from build123d import *

# Parameters (mm, degrees)
F0_W     = 75
F0_H     = 100
F0_R     = 4
F1_DEPTH = 2
F2_R     = 1.584077
F2_R_2   = 1.709737
F2_R_3   = 1.732285
F2_R_4   = 1.739733
F2_R_5   = 1.525849
F2_R_6   = 1.456457
F2_R_7   = 1.732284
F2_R_8   = 1.660922
F2_R_9   = 1.609722
F2_R_10  = 1.290227
F2_R_11  = 1.875683
F2_R_12  = 1.517347
F2_R_13  = 1.874836
F2_R_14  = 1.624248
F2_R_15  = 1.319184
F2_R_16  = 1.584076
F2_R_17  = 1.326308
F2_R_18  = 1.625082
F2_R_19  = 1.798229
F2_R_20  = 1.936752
F2_R_21  = 2.097076
F2_R_22  = 1.963284
F2_R_23  = 1.709734
F2_R_24  = 1.517348
F2_R_25  = 1.525848
F2_R_26  = 1.482857
F2_R_27  = 1.936751
F2_R_28  = 1.608384
F2_R_29  = 1.482858
F2_R_30  = 1.709736
F2_R_31  = 1.608385
F3_DEPTH = 1


with BuildPart() as f1:
    # F0 (on Top) → F1 (new body)
    with BuildSketch(Plane.XY):
        Rectangle(F0_W, F0_H)
        with Locations((-28.5, -41)):
            Circle(F0_R, mode=Mode.SUBTRACT)
        with Locations((-28.5, 41)):
            Circle(F0_R, mode=Mode.SUBTRACT)
    extrude(amount=F1_DEPTH)

    # F2 (on face) → F3 (join)
    with BuildSketch(Plane.XY.offset(2)):
        Polygon((-9.121194, -22.654161), (-9.121194, -33.186409), (0, -38.452533), (9.121194, -33.186409), (9.121194, -22.654161), (0, -17.388037), align=None)
        with Locations((28.836682, -14.088176)):
            Circle(F2_R)
        with Locations((34.787707, -10.549731)):
            Circle(F2_R_2)
        with Locations((34.466032, -5.724576)):
            Circle(F2_R_3)
        with Locations((29.480038, -5.563737)):
            Circle(F2_R_4)
        with Locations((25.298238, -7.654637)):
            Circle(F2_R_5)
        with Locations((18.864698, -13.60566)):
            Circle(F2_R_6)
        with Locations((14.039545, -8.29799)):
            Circle(F2_R_7)
        with Locations((19.82973, 0)):
            Circle(F2_R_8)
        with Locations((14.361222, 0)):
            Circle(F2_R_9)
        with Locations((8.410199, 0)):
            Circle(F2_R_10)
        with Locations((7.927684, -7.493799)):
            Circle(F2_R_11)
        with Locations((-9.442871, -11.997276)):
            Circle(F2_R_12)
        with Locations((0.046599, 0)):
            Circle(F2_R_13)
        with Locations((-7.351971, 0)):
            Circle(F2_R_14)
        with Locations((-13.946348, 0)):
            Circle(F2_R_15)
        with Locations((-18.771502, -5.402898)):
            Circle(F2_R_16)
        with Locations((-26.813426, -4.920383)):
            Circle(F2_R_12)
        with Locations((-13.946348, -11.675598)):
            Circle(F2_R_17)
        with Locations((-23.435817, 0)):
            Circle(F2_R_18)
        with Locations((-33.407803, 0)):
            Circle(F2_R_18)
        with Locations((-33.568642, -5.081222)):
            Circle(F2_R_12)
        with Locations((-9.121194, 10.198432)):
            Circle(F2_R_19)
        with Locations((-10.086225, 17.597001)):
            Circle(F2_R_20)
        with Locations((-7.351971, 22.904672)):
            Circle(F2_R_21)
        with Locations((11.626968, 23.065509)):
            Circle(F2_R_22)
        with Locations((14.36122, 30.946596)):
            Circle(F2_R_23)
        with Locations((14.039546, 36.254264)):
            Circle(F2_R_24)
        with Locations((19.347215, 42.04445)):
            Circle(F2_R_25)
        with Locations((7.28433, 42.04445)):
            Circle(F2_R_5)
        with Locations((1.976661, 36.254264)):
            Circle(F2_R_26)
        with Locations((-7.351971, 36.254264)):
            Circle(F2_R_27)
        with Locations((-13.946348, 36.254264)):
            Circle(F2_R_28)
        with Locations((-13.946348, 42.04445)):
            Circle(F2_R_29)
        with Locations((-18.932341, 42.04445)):
            Circle(F2_R_12)
        with Locations((-18.932341, 36.254264)):
            Circle(F2_R_16)
        with Locations((-23.918333, 36.254264)):
            Circle(F2_R_30)
        with Locations((-26.813426, 30.946596)):
            Circle(F2_R_26)
        with Locations((-26.813426, 18.079517)):
            Circle(F2_R_19)
        with Locations((-17.002279, 21.617964)):
            Circle(F2_R_31)
    extrude(amount=F3_DEPTH)


solid = f1.part
Read the model definition and answer for the solid it produces. Units are mm, in the model's axes. A direction names the side the tool comes from. Round coordinates to 2 decimals unless told otherwise and drop trailing zeros. Loops run counter-clockwise (first coordinate to the right, second up) from the corner with the lowest first, then second, coordinate; pieces in that order, holes last.
Q1. Consider probe 1 along Y at (x, z) = (-28.5, 1.5); probe 2 along Z at (x, y) = (21, -34.5); probe 3 along X at (y, z) = (-24, 2.65). Determine where each line is inside the solid, lowest interval first.
Q2. This flat-tipped pin is pushed along its axis until it touches: pin 1 (0.5 mm diameter, centred on y = -30.5, z = 2.5, fed in from +X). Where does it stop, or does it pass through?
Q3. Section A-A on y = -41 is taken. Write down the section's boundary in (x, z), and give its area (3 significant figures).
Q4. Determine the mould class of faces 1 (the face through (-12.577, 41.477, 2.493)), 2 (the face through (-22.3, 36.8, 2.5)), 3 (the face through (-4.624, -35.783, 2.493)), 4 (the face through (-33, 0, 3)) for opening direction Y: released by +Y, released by -Y, zero draft, split by the parting line, or undercut.
Q5. Which of the six approach directions +Z, -Z, +X, -X, +Y, -Y give full straight-line access (tool end or side, diameter ignored) to faces 5 (the face through (-28.61, 18.16, 2.49)), 6 (the face through (-4.497, -19.984, 2.493)), 7 (the face through (14, -8, 3))?
Q6. Section B-B on y = 26.5 is taken. Write down the section's boundary in (x, z), and give its area (3 significant figures).
Output:
1. probe 1: y = -50 to -45, -37 to 37, 45 to 50
1. probe 2: z = 0 to 2
1. probe 3: x = -9.12 to 9.12
2. pin 1: stops at x = 9.12
3. outline: (-37.5, 0) - (-32.5, 0) - (-32.5, 2) - (-37.5, 2) - close; (-24.5, 0) - (37.5, 0) - (37.5, 2) - (-24.5, 2) - close
3. area: 134 mm2
4. face 1: undercut
4. face 2: undercut
4. face 3: released by -Y
4. face 4: zero draft
5. face 5: +Z
5. face 6: +Z, -X
5. face 7: +Z, +X, -X, +Y, -Y
6. outline: (-37.5, 0) - (37.5, 0) - (37.5, 2) - (-37.5, 2) - close
6. area: 150 mm2
